Design review of the part built by this model. Coordinates are the model's own, in mm. Round coordinates to 2 decimals unless told otherwise and drop trailing zeros. Order: outer loops, then holes, each group sorted by start corner. A loop starts at its lowest first (then second) coordinate and runs counter-clockwise, first axis right, second up. Notation, with made-up numbers: M 48.5,66 L 104.5,66 A34 cw 104.5,100 Z; hole C 30,35.5 d5. An arc over 180 degrees is marked long. Write each question's results on one line, items separated by ' | '. Start each with the question number.
Item 1: Take a section at D-D, the plane y = 1.5. Count the separate pieces of the cut face and the enclosed holes in it, plus the area to 3 significant figures.
Item 2: Take a section at C-C, the plane z = 35.5. Write out the cut boundary in (x, y) (3 decimals).
Item 3: Wall thickness on line 1 (Z direction, x = 24, y = 5.5) (3 decimals); line 2 (X direction, y = 2.5, z = -41) (3 decimals); line 3 (Z direction, x = 51.5, y = 3) (3 decimals): over which ranges is each line inside the solid? List them lowest first. Write a range as [from, to].
Item 4: Clearance check with a flat-ended pin moving along its axis: pin 1 (10 mm diameter, centred on x = 48, z = 3.5, fed in from -Y). State where the tip first meets the part, or that it passes through.
Item 5: Take a section at A-A, the plane z = -44. Write out the cut boundary in (x, y) (3 decimals).
Item 6: Take a section at B-B, the plane x = 50. Write out the cut boundary in (y, z) (3 decimals), plus the area to 3 significant figures.
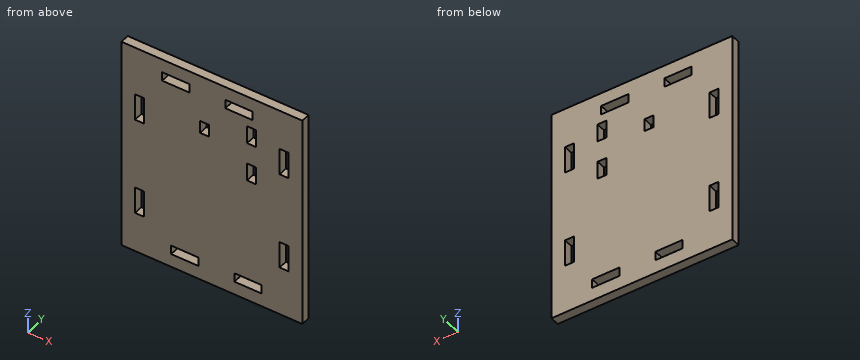
```python
from build123d import *

# Parameters (mm, degrees)
SKETCH1_W         = 127
SKETCH1_H         = 152.4
SKETCH1_W_2       = 19.05
SKETCH1_H_2       = 6.35
SKETCH1_W_3       = 6.35
SKETCH1_H_3       = 19.05
BASE_DEPTH        = 6.35
SKETCH2_W         = 6.35
SKETCH2_H         = 12.7
SKETCH2_H_2       = 8.89
MOTORMOUNTS_DEPTH = 100.3932216


with BuildPart() as part:
    # Sketch1 → BASE (new body)
    with BuildSketch(Plane(origin=(0, 0, 0), x_dir=(1, 0, 0), z_dir=(0, 1, 0))):
        Rectangle(SKETCH1_W, SKETCH1_H)
        with Locations((-19.05, 63.5)):
            Rectangle(SKETCH1_W_2, SKETCH1_H_2, mode=Mode.SUBTRACT)
        with Locations((25.4, 63.5)):
            Rectangle(SKETCH1_W_2, SKETCH1_H_2, mode=Mode.SUBTRACT)
        with Locations((-50.8, 38.1)):
            Rectangle(SKETCH1_W_3, SKETCH1_H_3, mode=Mode.SUBTRACT)
        with Locations((-50.8, -31.75)):
            Rectangle(SKETCH1_W_3, SKETCH1_H_3, mode=Mode.SUBTRACT)
        with Locations((-25.4, -63.5)):
            Rectangle(SKETCH1_W_2, SKETCH1_H_2, mode=Mode.SUBTRACT)
        with Locations((19.05, -63.5)):
            Rectangle(SKETCH1_W_2, SKETCH1_H_2, mode=Mode.SUBTRACT)
        with Locations((50.8, -38.1)):
            Rectangle(SKETCH1_W_3, SKETCH1_H_3, mode=Mode.SUBTRACT)
        with Locations((50.8, 31.75)):
            Rectangle(SKETCH1_W_3, SKETCH1_H_3, mode=Mode.SUBTRACT)
    extrude(amount=BASE_DEPTH)

    # Sketch2 → MOTORMOUNTS (cut, through all)
    with BuildSketch(Plane(origin=(0, 6.35, 0), x_dir=(1, 0, 0), z_dir=(0, 1, 0))):
        with Locations((27.94, -19.685)):
            Rectangle(SKETCH2_W, SKETCH2_H)
        with Locations((27.94, -47.625)):
            Rectangle(SKETCH2_W, SKETCH2_H)
        with Locations((-5.08, -38.1)):
            Rectangle(SKETCH2_W, SKETCH2_H_2)
    extrude(amount=-MOTORMOUNTS_DEPTH, mode=Mode.SUBTRACT)


solid = part.part
```
Results list:
1) separate pieces: 1 | enclosed holes: 11 | area: 18,200 mm²
2) outline: M -63.5,0 L -53.975,0 L -53.975,6.35 L -63.5,6.35 Z; M -47.625,0 L -8.255,0 L -8.255,6.35 L -47.625,6.35 Z; M -1.905,0 L 47.625,0 L 47.625,6.35 L -1.905,6.35 Z; M 53.975,0 L 63.5,0 L 63.5,6.35 L 53.975,6.35 Z
3) line 1: [-76.2, -66.675], [-60.325, 60.325], [66.675, 76.2] | line 2: [-63.5, -53.975], [-47.625, 47.625], [53.975, 63.5] | line 3: [-76.2, -41.275], [-22.225, 28.575], [47.625, 76.2]
4) pin 1: y = 0
5) outline: M -63.5,0 L -53.975,0 L -53.975,6.35 L -63.5,6.35 Z; M -47.625,0 L 63.5,0 L 63.5,6.35 L -47.625,6.35 Z
6) outline: M 0,-76.2 L 6.35,-76.2 L 6.35,-41.275 L 0,-41.275 Z; M 0,-22.225 L 6.35,-22.225 L 6.35,28.575 L 0,28.575 Z; M 0,47.625 L 6.35,47.625 L 6.35,76.2 L 0,76.2 Z | area: 726 mm²
